from build123d import *

# Parameters (mm, degrees)
SKETCH1_W           = 8.6
SKETCH1_H           = 27
BOSS_EXTRUDE1_DEPTH = 31.5
SKETCH2_W           = 27
SKETCH2_H           = 3
BOSS_EXTRUDE2_DEPTH = 40.5
SKETCH3_W           = 3
SKETCH3_H           = 28.5
BOSS_EXTRUDE3_DEPTH = 40.5
SKETCH4_W           = 8.6
SKETCH4_H           = 27
BOSS_EXTRUDE4_DEPTH = 31.5
CUT_EXTRUDE8_DEPTH  = 10
FILLET1_R           = 3
SKETCH5_R           = 2.2
CUT_EXTRUDE1_DEPTH  = 5
SKETCH6_W           = 17.5
SKETCH6_H           = 10
CUT_EXTRUDE2_DEPTH  = 10
FILLET3_R           = 1
SKETCH9_W           = 27
SKETCH9_H           = 5
BOSS_EXTRUDE5_DEPTH = 22.5
SKETCH10_R          = 2.2
CUT_EXTRUDE5_DEPTH  = 100
FILLET4_R           = 3
FILLET5_R           = 0.3
SKETCH12_W          = 14.05
SKETCH12_H          = 27
CUT_EXTRUDE6_DEPTH  = 10
FILLET6_R           = 3
SKETCH13_R          = 3.05
CUT_EXTRUDE7_DEPTH  = 10


with BuildPart() as part:
    # Sketch1 → Boss-Extrude1 (new body)
    with BuildSketch(Plane(origin=(0, 0, 0), x_dir=(1, 0, 0), z_dir=(0, 1, 0))):
        with Locations((4.3, 0)):
            Rectangle(SKETCH1_W, SKETCH1_H)
    extrude(amount=BOSS_EXTRUDE1_DEPTH)

    # Sketch2 → Boss-Extrude2 (add)
    with BuildSketch(Plane(origin=(8.6, 0, 0), x_dir=(0, 0, -1), z_dir=(1, 0, 0))):
        with Locations((0, 1.5)):
            Rectangle(SKETCH2_W, SKETCH2_H)
    extrude(amount=BOSS_EXTRUDE2_DEPTH)

    # Sketch3 → Boss-Extrude3 (add)
    with BuildSketch(Plane(origin=(8.6, 0, 0), x_dir=(0, 0, -1), z_dir=(1, 0, 0))):
        with Locations((12, 17.25)):
            Rectangle(SKETCH3_W, SKETCH3_H)
    extrude(amount=BOSS_EXTRUDE3_DEPTH)

    # Sketch4 → Boss-Extrude4 (add)
    with BuildSketch(Plane(origin=(0, 31.5, 0), x_dir=(1, 0, 0), z_dir=(0, 1, 0))):
        with Locations((53.4, 0)):
            Rectangle(SKETCH4_W, SKETCH4_H)
    extrude(amount=-BOSS_EXTRUDE4_DEPTH)

    # Sketch15 → Cut-Extrude8 (cut)
    with BuildSketch(Plane.XY.offset(-10.5)):
        with BuildLine():
            Line((31.35, 8.25), (31.35, 26.25))
            ThreePointArc((31.35, 26.25), (28.85, 28.75), (26.35, 26.25))
            Line((26.35, 26.25), (26.35, 8.25))
            ThreePointArc((26.35, 8.25), (28.85, 5.75), (31.35, 8.25))
        make_face()
        with BuildLine():
            Line((42.725, 8.25), (42.725, 26.25))
            ThreePointArc((42.725, 26.25), (40.225, 28.75), (37.725, 26.25))
            Line((37.725, 26.25), (37.725, 8.25))
            ThreePointArc((37.725, 8.25), (40.225, 5.75), (42.725, 8.25))
        make_face()
        with BuildLine():
            Line((19.975, 8.25), (19.975, 26.25))
            ThreePointArc((19.975, 26.25), (17.475, 28.75), (14.975, 26.25))
            Line((14.975, 26.25), (14.975, 8.25))
            ThreePointArc((14.975, 8.25), (17.475, 5.75), (19.975, 8.25))
        make_face()
    extrude(amount=-CUT_EXTRUDE8_DEPTH, mode=Mode.SUBTRACT)

    # Fillet1
    fillet1_edges = [part.edges().sort_by_distance(p)[0] for p in [
        (57.7, 15.75, -13.5),
        (57.7, 15.75, 13.5),
        (49.1, 17.25, 13.5),
        (8.6, 17.25, 13.5),
    ]]
    fillet(fillet1_edges, radius=FILLET1_R)

    # Sketch5 → Cut-Extrude1 (cut)
    with BuildSketch(Plane(origin=(0, 31.5, 0), x_dir=(1, 0, 0), z_dir=(0, 1, 0))):
        with Locations(Location((53.4, 4.95, 0), (0, 0, 270))):
            Circle(SKETCH5_R)
        with Locations(Location((53.4, -4.95, 0), (0, 0, 270))):
            Circle(SKETCH5_R)
        with Locations(Location((4.3, 4.95, 0), (0, 0, 270))):
            Circle(SKETCH5_R)
        with Locations(Location((4.3, -4.95, 0), (0, 0, 270))):
            Circle(SKETCH5_R)
    extrude(amount=-CUT_EXTRUDE1_DEPTH, mode=Mode.SUBTRACT)

    # Sketch6 → Cut-Extrude2 (cut)
    with BuildSketch(Plane.ZY.offset(-49.1)):
        with Locations((4.75, 10)):
            Rectangle(SKETCH6_W, SKETCH6_H)
    extrude(amount=-CUT_EXTRUDE2_DEPTH, mode=Mode.SUBTRACT)

    # Fillet3
    fillet3_edges = [part.edges().sort_by_distance(p)[0] for p in [
        (56.821320344, 5, 12.621320344),
        (56.821320344, 15, 12.621320344),
        (57.7, 10, -4),
        (49.1, 5, 3.25),
        (49.1, 15, 3.25),
        (49.1, 10, -4),
        (49.978679656, 15, 12.621320344),
        (57.7, 15, 3.25),
        (53.4, 15, 13.5),
        (49.978679656, 5, 12.621320344),
        (57.7, 5, 3.25),
        (53.4, 15, -4),
        (53.4, 5, 13.5),
        (53.4, 5, -4),
    ]]
    fillet(fillet3_edges, radius=FILLET3_R)

    # Sketch9 → Boss-Extrude5 (add)
    with BuildSketch(Plane.ZY):
        with Locations((0, 29)):
            Rectangle(SKETCH9_W, SKETCH9_H)
        with Locations((0, 2.5)):
            Rectangle(SKETCH9_W, SKETCH9_H)
    extrude(amount=BOSS_EXTRUDE5_DEPTH)

    # Sketch10 → Cut-Extrude5 (cut)
    with BuildSketch(Plane(origin=(0, 31.5, 0), x_dir=(1, 0, 0), z_dir=(0, 1, 0))):
        with Locations(Location((-5.3, 4.95, 0), (0, 0, 90))):
            Circle(SKETCH10_R)
        with Locations(Location((-5.3, -4.95, 0), (0, 0, 90))):
            Circle(SKETCH10_R)
        with Locations(Location((-17.2, -4.95, 0), (0, 0, 90))):
            Circle(SKETCH10_R)
        with Locations(Location((-17.2, 4.95, 0), (0, 0, 90))):
            Circle(SKETCH10_R)
    extrude(amount=-CUT_EXTRUDE5_DEPTH, mode=Mode.SUBTRACT)

    # Fillet4
    fillet4_edges = [part.edges().sort_by_distance(p)[0] for p in [
        (0, 15.75, 13.5),
        (0, 15.75, -13.5),
        (-22.5, 2.5, 13.5),
        (-22.5, 2.5, -13.5),
    ]]
    fillet(fillet4_edges, radius=FILLET4_R)

    # Fillet5
    # the kernel refuses this fillet: 0.3 mm, written as the material it adds along each edge
    with BuildSketch(Plane(origin=(0, 5, 10.5), x_dir=(0, 1, 0), z_dir=(0, 0, -1))) as fillet5_piece_1:
        with BuildLine():
            CenterArc((FILLET5_R, -FILLET5_R), FILLET5_R, 90, 90)
            Line((0, -FILLET5_R), (0, 0))
            Line((0, 0), (FILLET5_R, 0))
        make_face()
    extrude(amount=21)
    with BuildSketch(Plane(origin=(0, 26.5, 10.5), x_dir=(0, -1, 0), z_dir=(0, 0, -1))) as fillet5_piece_2:
        with BuildLine():
            CenterArc((FILLET5_R, FILLET5_R), FILLET5_R, 180, 90)
            Line((0, FILLET5_R), (0, 0))
            Line((0, 0), (FILLET5_R, 0))
        make_face()
    extrude(amount=21)
    with BuildSketch(Plane(origin=(3, 5, -10.5), x_dir=(-1, 0, 0), z_dir=(0, 0, 1))) as fillet5_piece_3_section:
        with BuildLine():
            CenterArc((3 + FILLET5_R, -FILLET5_R), FILLET5_R, 90, 90)
            Line((3 + FILLET5_R, 0), (3, 0))
            Line((3, 0), (3, -FILLET5_R))
        make_face()
    fillet5_piece_3 = revolve(axis=Axis((3, 5, -10.5), (0, -1, 0)), revolution_arc=104.329698924, mode=Mode.PRIVATE)
    fillet5_piece_3 = split(fillet5_piece_3, bisect_by=Plane(origin=(0.81861369, 5.084946104, -13.5), z_dir=(0, 0, 1)), keep=Keep.TOP, mode=Mode.PRIVATE)
    add(fillet5_piece_3)
    with BuildSketch(Plane(origin=(3, 26.5, -10.5), x_dir=(-1, 0, 0), z_dir=(0, 0, 1))) as fillet5_piece_4_section:
        with BuildLine():
            CenterArc((3 + FILLET5_R, FILLET5_R), FILLET5_R, 180, 90)
            Line((3 + FILLET5_R, 0), (3, 0))
            Line((3, 0), (3, FILLET5_R))
        make_face()
    fillet5_piece_4 = revolve(axis=Axis((3, 26.5, -10.5), (0, -1, 0)), revolution_arc=104.329698924, mode=Mode.PRIVATE)
    fillet5_piece_4 = split(fillet5_piece_4, bisect_by=Plane(origin=(0.81861369, 26.415053896, -13.5), z_dir=(0, 0, 1)), keep=Keep.TOP, mode=Mode.PRIVATE)
    add(fillet5_piece_4)
    with BuildSketch(Plane(origin=(3, 5, 10.5), x_dir=(0.24750126301206385, 0, 0.968887570777659), z_dir=(0.968887570777659, 0, -0.24750126301206385))) as fillet5_piece_5_section:
        with BuildLine():
            CenterArc((3 + FILLET5_R, -FILLET5_R), FILLET5_R, 90, 90)
            Line((3 + FILLET5_R, 0), (3, 0))
            Line((3, 0), (3, -FILLET5_R))
        make_face()
    fillet5_piece_5 = revolve(axis=Axis((3, 5, 10.5), (0, -1, 0)), revolution_arc=104.329698924, mode=Mode.PRIVATE)
    fillet5_piece_5 = split(fillet5_piece_5, bisect_by=Plane(origin=(0.818613701, 5.084946089, 13.5), z_dir=(0, 0, -1)), keep=Keep.TOP, mode=Mode.PRIVATE)
    add(fillet5_piece_5)
    with BuildSketch(Plane(origin=(3, 26.5, 10.5), x_dir=(0.24750126301206454, 0, 0.9688875707776589), z_dir=(0.9688875707776589, 0, -0.24750126301206454))) as fillet5_piece_6_section:
        with BuildLine():
            CenterArc((3 + FILLET5_R, FILLET5_R), FILLET5_R, 180, 90)
            Line((3, FILLET5_R), (3, 0))
            Line((3, 0), (3 + FILLET5_R, 0))
        make_face()
    fillet5_piece_6 = revolve(axis=Axis((3, 26.5, 10.5), (0, -1, 0)), revolution_arc=104.329698924, mode=Mode.PRIVATE)
    fillet5_piece_6 = split(fillet5_piece_6, bisect_by=Plane(origin=(0.818613746, 26.41505391, 13.5), z_dir=(0, 0, -1)), keep=Keep.TOP, mode=Mode.PRIVATE)
    add(fillet5_piece_6)

    # Sketch12 → Cut-Extrude6 (cut)
    with BuildSketch(Plane(origin=(0, 31.5, 0), x_dir=(1, 0, 0), z_dir=(0, 1, 0))):
        with Locations((-15.475, 0)):
            Rectangle(SKETCH12_W, SKETCH12_H)
    extrude(amount=-CUT_EXTRUDE6_DEPTH, mode=Mode.SUBTRACT)

    # Fillet6
    fillet6_edges = [part.edges().sort_by_distance(p)[0] for p in [
        (-8.45, 29, -13.5),
        (-8.45, 29, 13.5),
    ]]
    fillet(fillet6_edges, radius=FILLET6_R)

    # Sketch13 → Cut-Extrude7 (cut)
    with BuildSketch(Plane.XZ):
        with Locations(Location((40.02, 0, 0), (0, 0, 270))):
            Circle(SKETCH13_R)
    extrude(amount=-CUT_EXTRUDE7_DEPTH, mode=Mode.SUBTRACT)


solid = part.part
Verification items for the finished model (mm, model axes). A direction names the side the tool comes from. Give positions to 0.01 mm unless a question says otherwise; leave off trailing zeros. Write each loop counter-clockwise with the first axis right and the second up, starting at its lowest first coordinate (ties: lowest second). Pieces come first, ordered by that corner, then holes. Notation, with made-up numbers: (2, 38.25) - (12, 38.25) arc R24 cw to (12, 52.25) - close; hole circle Ø1 at (21.5, 34.25). An arc over 180 degrees is marked (long way). Answer as CSV lines item,"result". Start each with the question number.
1. Sectioned sample at C-C (x = -17.2). Record the boundary of the cut face in (y, z), then the cut area to 3 significant figures.
2. Sectioned sample at A-A (z = 9.5). Record the boundary of the cut face in (x, y), then the cut area to 3 significant figures.
3. Depth check by flat-ended pin: pin 1 (1.3 mm diameter, centred on x = 4.5, z = 5.5, fed in from +Y); pin 2 (5.5 mm diameter, centred on x = 54, y = 9.5, fed in from +Z); pin 3 (2.5 mm diameter, centred on y = 19.5, z = -11.5, fed in from -X); pin 4 (1 mm diameter, centred on x = 27.5, y = 12.5, fed in from +Z). Enter the tip coordinate at first touch or a pass-through.
4. Thickness scan on line 1 (X direction, y = 3.5, z = -4.95); line 2 (X direction, y = 29.8, z = -4.95); line 3 (X direction, y = 2.6, z = -4.95). Record the ranges inside material, lowest first.
5. Draft check along X on faces 1 (the face through (25, 31.5, -11)), 2 (the face through (33, 17, -10.5)), 3 (the face through (-8.45, 29, 0)). Enter one of: pulls with the +X half, pulls with the -X half, needs draft (parallel to the pull), parting line crosses it, or undercut.
6. Sectioned sample at D-D (y = 24). Record the boundary of the cut face in (x, z) (3 decimals), then the cut area to 3 significant figures.
7. Sectioned sample at B-B (z = 0). Record the boundary of the cut face in (x, y), then the cut area to 3 significant figures.
8. Set-up check for faces 4 (the face through (4, 26.5, 5)), 5 (the face through (0, 16, 0)), 6 (the face through (29, 3, 2)), 7 (the face through (40.17, 5.75, -11.98)): record each of +Z, -Z, +X, -X, +Y, -Y from which the full face is reachable in a straight line by a thin tool's end or side.
Derived:
1,outline,"(0, -13.5) - (5, -13.5) - (5, -7.15) - (0, -7.15) - close; (0, -2.75) - (5, -2.75) - (5, 2.75) - (0, 2.75) - close; (0, 7.15) - (5, 7.15) - (5, 13.5) - (0, 13.5) - close"
1,area,"91.0 mm²"
2,outline,"(-22.5, 0) - (57.7, 0) - (57.7, 4) arc R1 ccw to (56.7, 5) - (50.1, 5) arc R1 ccw to (49.1, 4) - (49.1, 3) - (8.6, 3) - (8.6, 31.5) - (-8.45, 31.5) - (-8.45, 26.5) - (-0.3, 26.5) arc R0.3 cw to (0, 26.2) - (0, 5.3) arc R0.3 cw to (-0.3, 5) - (-22.5, 5) - close; (49.1, 16) arc R1 ccw to (50.1, 15) - (56.7, 15) arc R1 ccw to (57.7, 16) - (57.7, 31.5) - (49.1, 31.5) - close"
2,area,"731 mm²"
3,pin 1,"y = 26.5"
3,pin 2,"z = -4"
3,pin 3,"x = 0"
3,pin 4,"through"
4,line 1,"-22.5 to -19.4, -15 to -7.5, -3.1 to 8.6, 49.1 to 57.7"
4,line 2,"-8.45 to -7.5, -3.1 to 2.1, 6.5 to 8.6, 49.1 to 51.2, 55.6 to 57.7"
4,line 3,"-22.5 to -19.4, -15 to -7.5, -3.1 to 57.7"
5,face 1,"needs draft"
5,face 2,"undercut"
5,face 3,"pulls with the -X half"
6,outline,"(0, -10.5) arc R3 ccw to (3, -13.5) - (14.975, -13.5) - (14.975, -10.5) - (8.6, -10.5) - (8.6, 10.5) arc R3 ccw to (5.6, 13.5) - (3, 13.5) arc R3 ccw to (0, 10.5) - close; (19.975, -13.5) - (26.35, -13.5) - (26.35, -10.5) - (19.975, -10.5) - close; (31.35, -13.5) - (37.725, -13.5) - (37.725, -10.5) - (31.35, -10.5) - close; (42.725, -13.5) - (54.7, -13.5) arc R3 ccw to (57.7, -10.5) - (57.7, 10.5) arc R3 ccw to (54.7, 13.5) - (52.1, 13.5) arc R3 ccw to (49.1, 10.5) - (49.1, -10.5) - (42.725, -10.5) - close"
6,area,"529 mm²"
7,outline,"(-22.5, 0) - (36.97, 0) - (36.97, 3) - (8.6, 3) - (8.6, 31.5) - (-8.45, 31.5) - (-8.45, 26.5) - (-0.3, 26.5) arc R0.3 cw to (0, 26.2) - (0, 5.3) arc R0.3 cw to (-0.3, 5) - (-22.5, 5) - close; (43.07, 0) - (57.7, 0) - (57.7, 4) arc R1 ccw to (56.7, 5) - (50.1, 5) arc R1 ccw to (49.1, 4) - (49.1, 3) - (43.07, 3) - close; (49.1, 16) arc R1 ccw to (50.1, 15) - (56.7, 15) arc R1 ccw to (57.7, 16) - (57.7, 31.5) - (49.1, 31.5) - close"
7,area,"713 mm²"
8,face 4,"+Y"
8,face 5,"+Z, -Z, -X"
8,face 6,"+Z, +Y"
8,face 7,"+Z, -Z"
